The model under review builds one solid part; all positions refer to its coordinate system, in mm. Face numbers are marked on the shaded views. A direction names the side the tool comes from. Round coordinates to 2 decimals unless told otherwise and drop trailing zeros. Order: outer loops, then holes, each group sorted by start corner. A loop starts at its lowest first (then second) coordinate and runs counter-clockwise, first axis right, second up. Notation, with made-up numbers: (-16.5, 11.5) -> (-0.5, 11.5) arc R24 ccw to (-0.5, 48.5) -> close; hole circle Ø7 at (-25.5, -37.75). An arc over 180 degrees is marked (long way). Use a Markdown table: item, result. Add a question column.
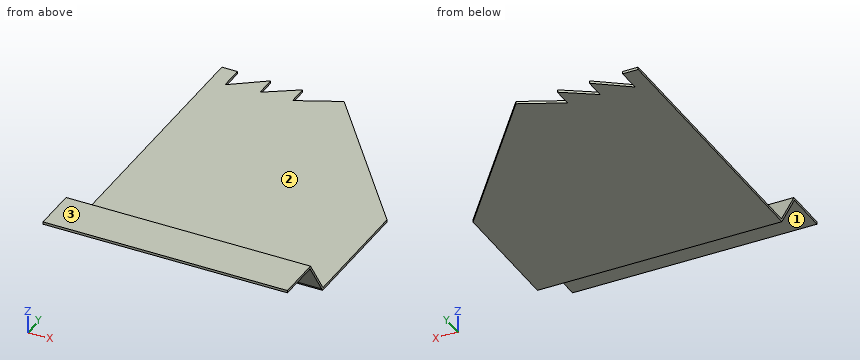
```python
from build123d import *

# Parameters (mm, degrees)
F1_DEPTH = 100
F3_DEPTH = 25


with BuildPart() as f1:
    # F0 (on Right) → F1 (new body)
    with BuildSketch(Plane.YZ):
        Polygon((75, 0.5), (-38.848786, 0.5), (-48.764013, 15.543181), (-67.072637, 15.543181), (-67.072637, 14.543181), (-49.104895, 14.543181), (-39.848786, 0.5), (-39.189668, -0.5), (75, -0.5), align=None)
    extrude(amount=F1_DEPTH)

    # F2 (on face) → F3 (cut)
    with BuildSketch(Plane.XY.offset(0.5)):
        Polygon((33.065695, 66.954866), (50, 75), (33.065695, 75), align=None)
        Polygon((19.983491, 66.483282), (33.065695, 75), (19.983491, 75), align=None)
        Polygon((6.371066, 65.092333), (19.983491, 75), (6.371066, 75), align=None)
        Polygon((50, 75), (100, 12.005576), (100, 75), align=None)
        Polygon((100, 75), (100, 12.005576), (155.00921, 119.249597), (16.864885, 99.318206), (6.371066, 75), (19.983491, 75), (33.065695, 75), (50, 75), align=None)
    extrude(amount=-F3_DEPTH, mode=Mode.SUBTRACT)


solid = f1.part
```
Q1. To check wall thickness, follow line 1 along Z through (x, y) = (56, 60); line 2 along Y through (x, z) = (82, 1.5); line 3 along Y through (x, z) = (55, 8.25). State the ranges of each line that lie inside material, in increasing order.
Q2. Add section C-C, the plane x = 13. Give the boundary of the cut face in (y, z), then the cut area to 3 significant figures.
Q3. Add section D-D, the plane z = 7. Give the boundary of the cut face in (x, y).
Q4. For the marked faces 1, 2 and 3, list the 3-axis set-ups (+Z, -Z, +X, -X, +Y, -Y) from which the entire face can be reached by the end or side of a thin tool; tool diameter is ignored.
Q5. For pin 1 (1 mm diameter, centred on x = 71, z = 13, fed in from -Y); pin 2 (0.5 mm diameter, centred on y = 71.5, z = 0, fed in from +X); pin 3 (0.8 mm diameter, centred on y = 71, z = 0, fed in from +X), all flat-tipped, find the tip position at first contact; note any pin that passes through.
Q6. Add section B-B, the plane y = -8. Give the boundary of the cut face in (x, z).
Q7. Add section A-A, the plane x = 84. Give the boundary of the cut face in (y, z).
Return value:
| question | item | result |
|---|---|---|
| 1 | line 1 | -0.5 to 0.5 |
| 1 | line 2 | -40.51 to -39.51 |
| 1 | line 3 | -44.96 to -43.96 |
| 2 | outline | (-67.07, 14.54) -> (-49.1, 14.54) -> (-39.85, 0.5) -> (-39.19, -0.5) -> (69.92, -0.5) -> (69.92, 0.5) -> (-38.85, 0.5) -> (-48.76, 15.54) -> (-67.07, 15.54) -> close |
| 2 | area | 142 mm² |
| 3 | outline | (0, -44.13) -> (100, -44.13) -> (100, -43.13) -> (0, -43.13) -> close |
| 4 | face 1 | -Z, +X, -X, -Y |
| 4 | face 2 | +Z, +X, -X, +Y |
| 4 | face 3 | +Z, +X, -X, +Y, -Y |
| 5 | pin 1 | y = -48.42 |
| 5 | pin 2 | x = 52.98 |
| 5 | pin 3 | x = 53.49 |
| 6 | outline | (0, -0.5) -> (100, -0.5) -> (100, 0.5) -> (0, 0.5) -> close |
| 7 | outline | (-67.07, 14.54) -> (-49.1, 14.54) -> (-39.85, 0.5) -> (-39.19, -0.5) -> (32.16, -0.5) -> (32.16, 0.5) -> (-38.85, 0.5) -> (-48.76, 15.54) -> (-67.07, 15.54) -> close |
